The drawing under review shows one solid part. Ordinate dimensions are in mm from its lowest x, y, z. Coordinates: 2 decimals unless noted, no trailing zeros. Order: outer loops, then holes, each group sorted by start corner. A loop starts at its lowest first (then second) coordinate and runs counter-clockwise, first axis right, second up. Notation, with made-up numbers: (-31, 23.25) -> (28, 23.25) arc R22 ccw to (28, 47.25) -> close; hole circle Ø8 at (-0.5, -37.75). An arc over 180 degrees is marked (long way). Write item = value, one per line.
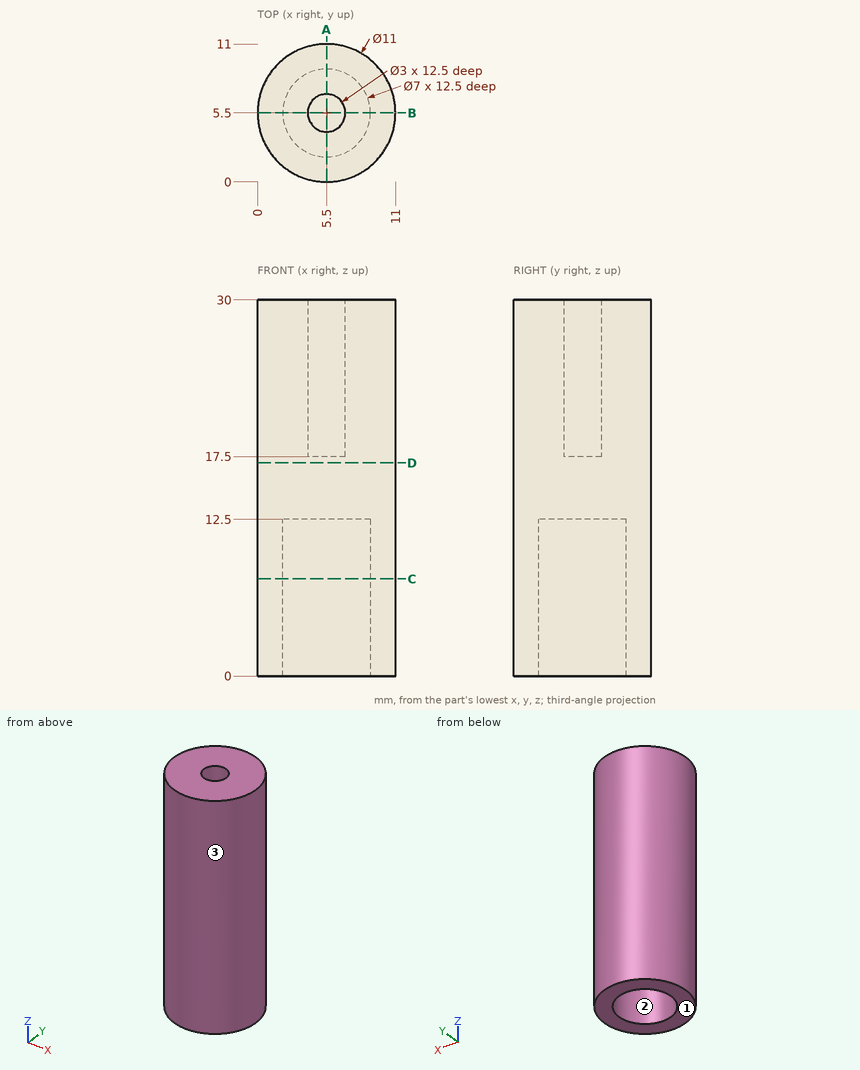
(1) For L1, parallel to Y at x = 5.5, z = 4.25; L2, parallel to Y at x = 5.25, z = 21.75; L3, parallel to X at y = 2.5, z = 9.75, list the stretches that pass through material, from the lowest coordinate up.
Report:
L1 = 0 to 2, 9 to 11
L2 = 0.01 to 4.02, 6.98 to 10.99
L3 = 0.89 to 3.7, 7.3 to 10.11
(2) We need section D-D (z = 17). Write out the cut boundary in (x, y).
Report:
outline = circle Ø11 at (5.5, 5.5)
(3) Insertion check: pin 1 (2 mm diameter, centred on x = 8.5, z = 10, fed in from -Y); pin 2 (3.5 mm diameter, centred on x = 7, y = 6, fed in from -Z); pin 3 (1.5 mm diameter, centred on x = 5.5, y = 5, fed in from +Z). Each pin has a flat end and moves straight along its axis. Give the tip position at first contact, or say it passes through.
Report:
pin_1 = 0.38
pin_2 = 12.5
pin_3 = 17.5
(4) The part is to be moulded in two halves that separate along X. For the marked faces 1, 2 and 3, say which applies: released by +X, released by -X, zero draft, split by the parting line, or undercut.
Report:
face_1 = zero draft
face_2 = undercut
face_3 = split by the parting line
(5) We need section A-A (x = 5.5). Write out the cut boundary in (y, z), and give its area (3 significant figures).
Report:
outline = (0, 0) -> (2, 0) -> (2, 12.5) -> (9, 12.5) -> (9, 0) -> (11, 0) -> (11, 30) -> (7, 30) -> (7, 17.5) -> (4, 17.5) -> (4, 30) -> (0, 30) -> close
area = 205 mm²
(6) We need section C-C (z = 7.75). Write out the cut boundary in (x, y), and give its area (3 significant figures).
Report:
outline = circle Ø11 at (5.5, 5.5); hole circle Ø7 at (5.5, 5.5)
area = 56.5 mm²
